Part print with two shaded views. Sizes in mm from the minimum x, y, z corner. A direction names the side the tool comes from. Give positions to 0.01 mm unless a question says otherwise; leave off trailing zeros. Write each loop counter-clockwise with the first axis right and the second up, starting at its lowest first coordinate (ties: lowest second). Pieces come first, ordered by that corner, then holes.
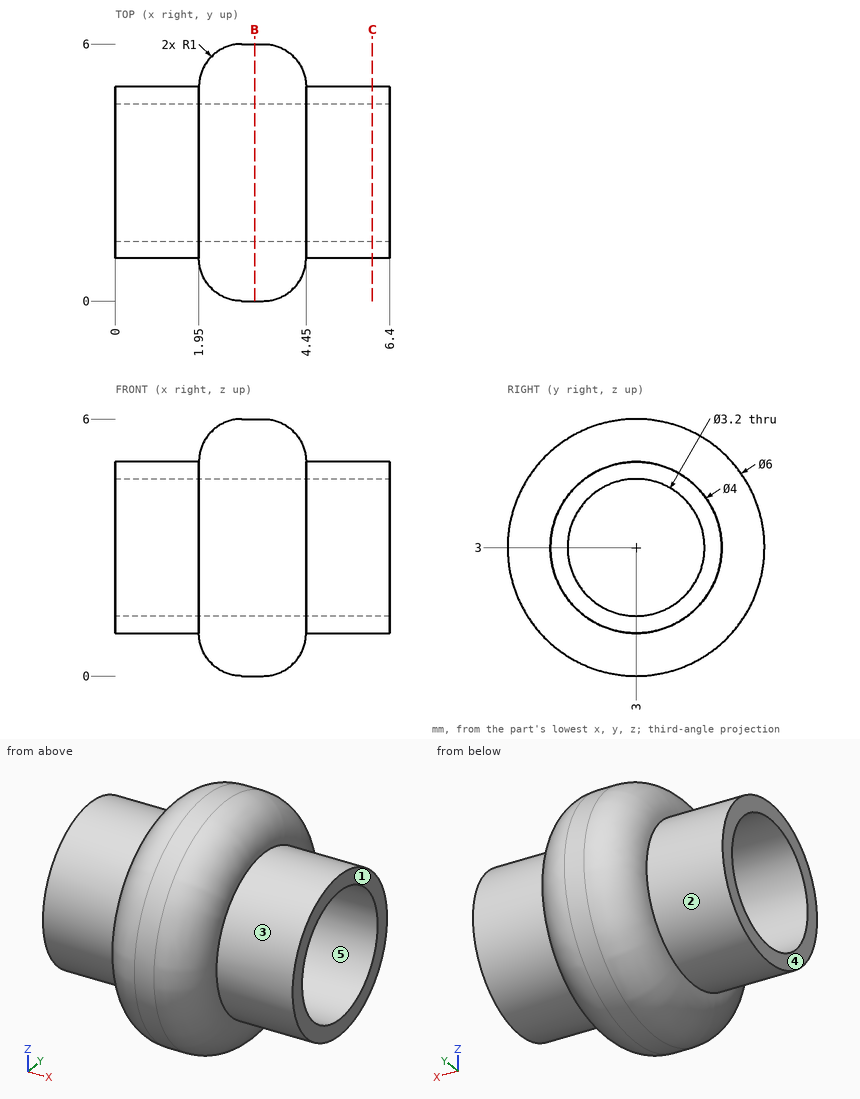
1) 3-axis set-ups, long thin cutter, end or side, ignore diameter. For the marked faces 1 and 2: which of +Z, -Z, +X, -X, +Y, -Y reach the whole face in a straight line?
Check result:
face 1: +Z, -Z, +X, +Y, -Y
face 2: -X
2) Saw through at C-C (x = 6). Write the cut outline in (y, z).
Check result:
outline: circle Ø4 at (3, 3); hole circle Ø3.2 at (3, 3)
3) Mould opens along Z. For the marked faces 3, 4 and 5 say: +Z half, -Z half, draft (parallel to the pull), parting line (faces both ways), or undercut.
Check result:
face 3: parting line
face 4: draft
face 5: undercut
4) Saw through at B-B (x = 3.25). Write the cut outline in (y, z), and give its area (3 significant figures).
Check result:
outline: circle Ø6 at (3, 3); hole circle Ø3.2 at (3, 3)
area: 20.2 mm2
5) Drill centre lines: L1, parallel to Y at x = 3.25, z = 3; L2, parallel to Y at x = 5.5, z = 1.6 (1 decimal); L3, parallel to Z at x = 2.25, y = 4. Where is each one in solid material? Low to high.
Check result:
L1: y = 0 to 1.4, 4.6 to 6
L2: y = 1.6 to 2.2, 3.8 to 4.4
L3: z = 0.48 to 1.75, 4.25 to 5.52
6) Flat gauge pins, fed straight in: P1, Ø1.9, axis at y = 3, z = 3, coming from the +X side; P2, Ø1, axis at x = 2.5, y = 2, coming from the +Z side; P3, Ø1, axis at x = 3.5, y = 2, coming from the +Z side. Where does each tip first touch, or does it go through?
Check result:
P1: passes through
P2: stops at z = 5.93
P3: stops at z = 5.96
